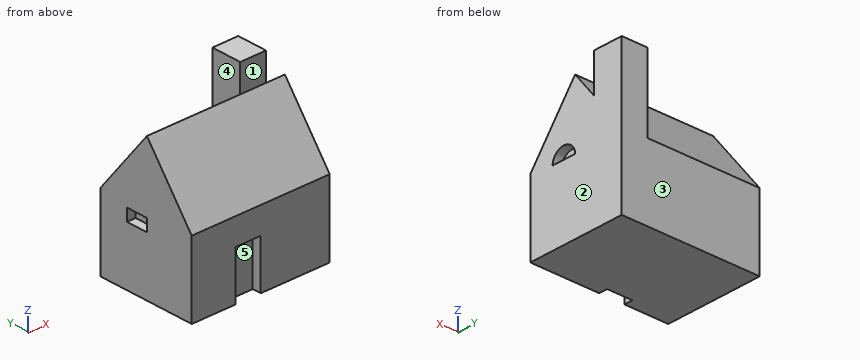
```python
from build123d import *

# Parameters (mm, degrees)
F1_DEPTH      = 50.8
F1_DEPTH_BACK = 50.8
F3_DEPTH      = 19.05
F4_W          = 18.4178259224
F4_H          = 35.4467518628
F5_DEPTH      = 6.35
F6_W          = 15.8175062388
F6_H          = 8.841086179
F7_DEPTH      = 6.35
F9_DEPTH      = 6.35


with BuildPart() as f1:
    # F0 (on Right) → F1 (new body, two sides)
    with BuildSketch(Plane.YZ) as f1_sk:
        Polygon((-35.6828793883, 54.4758699834), (-35.6828793883, 0), (37.1101982892, 0), (37.1101982892, 54.4758699834), (0, 101.5772745013), align=None)
    extrude(amount=F1_DEPTH)
    extrude(f1_sk.sketch, amount=-F1_DEPTH_BACK)

    # F2 (on face) → F3 (join)
    with BuildSketch(Plane.YZ.offset(50.8)):
        Polygon((14.9918657955, 110.3359609842), (14.9918657955, 82.5491375506), (37.1101982892, 54.4758699834), (37.1101982892, 110.3359609842), align=None)
    extrude(amount=-F3_DEPTH)

    # F4 (on face) → F5 (cut)
    with BuildSketch(Plane.XZ.offset(35.6828793883)):
        with Locations((-9.2089129612, 17.7233759314)):
            Rectangle(F4_W, F4_H)
    extrude(amount=-F5_DEPTH, mode=Mode.SUBTRACT)

    # F6 (on face) → F7 (cut)
    with BuildSketch(Plane(origin=(-50.8, 0, 0), x_dir=(0, -1, 0), z_dir=(-1, 0, 0))):
        with Locations((-7.9087531194, 46.6281268746)):
            Rectangle(F6_W, F6_H)
    extrude(amount=-F7_DEPTH, mode=Mode.SUBTRACT)

    # F8 (on face) → F9 (cut)
    with BuildSketch(Plane.YZ.offset(50.8)):
        with BuildLine():
            Line((-17.8977604955, 52.6088625193), (0, 52.6088625193))
            ThreePointArc((0, 52.6088625193), (-8.9488802478, 61.4720002386), (-17.8977604955, 52.6088625193))
        make_face()
    extrude(amount=-F9_DEPTH, mode=Mode.SUBTRACT)


solid = f1.part
```
Can you work these out from the model? Positions are in its coordinate system, mm. Face numbers are marked on the shaded views. A direction names the side the tool comes from. Round coordinates to 2 decimals unless told otherwise and drop trailing zeros. Loops run counter-clockwise (first coordinate to the right, second up) from the corner with the lowest first, then second, coordinate; pieces in that order, holes last. Notation, with made-up numbers: M 28,31.5 L 64,31.5 A24 cw 64,50.5 Z; hole C 37.25,19.25 d3. An arc over 180 degrees is marked long. Answer in a Markdown table with one row per item.
1. Please list where these lines run through material, in increasing order: line 1 (Y direction, x = -14, z = 24); line 2 (X direction, y = 16, z = 94.5); line 3 (X direction, y = -5, z = 60). Write a range as from..to.
Established:
| item | result |
|---|---|
| line 1 | -29.33..37.11 |
| line 2 | 31.75..50.8 |
| line 3 | -50.8..44.45 |
2. Thinking about a two-plate mould opening in X: for the marked faces 3, 4 and 5, which applies, pulls with the +X half, pulls with the -X half, needs draft (parallel to the pull), parting line crosses it, or undercut?
Established:
| item | result |
|---|---|
| face 3 | needs draft |
| face 4 | pulls with the -X half |
| face 5 | undercut |
3. If we section it at A-A, the plane z = 98.5: Please give me the cut outline in (x, y), plus the area to 3 significant figures.
Established:
| item | result |
|---|---|
| outline | M -50.8,-2.33 L 50.8,-2.33 L 50.8,2.42 L -50.8,2.42 Z; M 31.75,14.99 L 50.8,14.99 L 50.8,37.11 L 31.75,37.11 Z |
| area | 905 mm² |
4. If we section it at B-B, the plane x = -6: Please give me the cut outline in (y, z).
Established:
| item | result |
|---|---|
| outline | M -35.68,35.45 L -29.33,35.45 L -29.33,0 L 37.11,0 L 37.11,54.48 L 0,101.58 L -35.68,54.48 Z |
5. On a 3-axis mill with a long thin cutter (end or side, diameter ignored), from which of +Z, -Z, +X, -X, +Y, -Y can I reach the whole of each face in a straight line? I mean the marked faces 1 and 2. Say none if no direction works.
Established:
| item | result |
|---|---|
| face 1 | +Z, +X, -X |
| face 2 | +Z, -Z, +X, +Y, -Y |
6. If we section it at C-C, the plane z = 25: Please give me the cut outline in (x, y), plus the area to 3 significant figures.
Established:
| item | result |
|---|---|
| outline | M -50.8,-35.68 L -18.42,-35.68 L -18.42,-29.33 L 0,-29.33 L 0,-35.68 L 50.8,-35.68 L 50.8,37.11 L -50.8,37.11 Z |
| area | 7,280 mm² |
7. I'm going to push flat-ended pins straight in: pin 1 Ø1.9 at (x, y) = (-6, -34) entering from -Z; pin 2 Ø6 at (x, y) = (40.5, 6) entering from -Z; pin 3 Ø3 at (x, y) = (46.5, -12.5) entering from +Z; pin 4 Ø12 at (x, z) = (10, 97.5) entering from -Y. Where does each tip first touch, or does it pass through?
Established:
| item | result |
|---|---|
| pin 1 | z = 35.45 |
| pin 2 | z = 0 |
| pin 3 | z = 87.06 |
| pin 4 | y = -7.63 |
8. If we section it at D-D, the plane y = 21: Please give me the cut outline in (x, z).
Established:
| item | result |
|---|---|
| outline | M -50.8,0 L 50.8,0 L 50.8,110.34 L 31.75,110.34 L 31.75,74.92 L -50.8,74.92 Z |
